from build123d import *

# Parameters (mm, degrees)
SKETCH2_W           = 86.2
SKETCH2_H           = 20
SKETCH2_R           = 7
BOSS_EXTRUDE1_DEPTH = 45
SKETCH3_R           = 1.375
CUT_EXTRUDE1_DEPTH  = 66.441653402
SKETCH4_R           = 4
CUT_EXTRUDE2_DEPTH  = 17
SKETCH5_R           = 7
SKETCH5_R_2         = 5
BOSS_EXTRUDE2_DEPTH = 21
SKETCH6_R           = 2
SKETCH6_R_2         = 2.5
CUT_EXTRUDE3_DEPTH  = 66.441653402
SKETCH7_R           = 5
CUT_EXTRUDE4_DEPTH  = 16
CUT_EXTRUDE5_REACH  = 67.442
SKETCH8_R           = 1
SKETCH9_W           = 60
SKETCH9_H           = 24.2
CUT_EXTRUDE6_DEPTH  = 66.441653471


with BuildPart() as part:
    # Sketch2 → Boss-Extrude1 (new, symmetric)
    with BuildSketch(Plane(origin=(0, 0, 0), x_dir=(0, 0, -1), z_dir=(1, 0, 0))):
        Rectangle(SKETCH2_W, SKETCH2_H)
        with Locations(Location((-24.1, 0, 0), (0, 0, 180))):
            Circle(SKETCH2_R, mode=Mode.SUBTRACT)
        with Locations(Location((24.1, 0, 0), (0, 0, 180))):
            Circle(SKETCH2_R, mode=Mode.SUBTRACT)
    extrude(amount=BOSS_EXTRUDE1_DEPTH, both=True)

    # Sketch3 → Cut-Extrude1 (cut, through all)
    with BuildSketch(Plane.XZ.offset(10)):
        with Locations(Location((-38.1, 36.195, 0), (0, 0, 270))):
            Circle(SKETCH3_R)
        with Locations(Location((38.1, 36.195, 0), (0, 0, 270))):
            Circle(SKETCH3_R)
        with Locations(Location((38.1, -36.195, 0), (0, 0, 270))):
            Circle(SKETCH3_R)
        with Locations(Location((-38.1, -36.195, 0), (0, 0, 270))):
            Circle(SKETCH3_R)
    extrude(amount=-CUT_EXTRUDE1_DEPTH, mode=Mode.SUBTRACT)

    # Sketch4 → Cut-Extrude2 (cut)
    with BuildSketch(Plane(origin=(0, 10, 0), x_dir=(1, 0, 0), z_dir=(0, 1, 0))):
        with Locations(Location((-38.1, -36.195, 0), (0, 0, 270))):
            Circle(SKETCH4_R)
        with Locations(Location((-38.1, 36.195, 0), (0, 0, 270))):
            Circle(SKETCH4_R)
        with Locations(Location((38.1, 36.195, 0), (0, 0, 270))):
            Circle(SKETCH4_R)
        with Locations(Location((38.1, -36.195, 0), (0, 0, 270))):
            Circle(SKETCH4_R)
    extrude(amount=-CUT_EXTRUDE2_DEPTH, mode=Mode.SUBTRACT)

    # Sketch5 → Boss-Extrude2 (add, symmetric)
    # profile 1 of 2: a face of its own
    with BuildSketch(Plane(origin=(0, 0, 0), x_dir=(0, 0, -1), z_dir=(1, 0, 0))):
        with Locations(Location((24.1, 0, 0), (0, 0, 180))):
            Circle(SKETCH5_R)
        with Locations(Location((24.1, 0, 0), (0, 0, 180))):
            Circle(SKETCH5_R_2, mode=Mode.SUBTRACT)
    # profile 2 of 2: a face of its own
    with BuildSketch(Plane(origin=(0, 0, 0), x_dir=(0, 0, -1), z_dir=(1, 0, 0))):
        with Locations(Location((-24.1, 0, 0), (0, 0, 180))):
            Circle(SKETCH5_R)
        with Locations(Location((-24.1, 0, 0), (0, 0, 180))):
            Circle(SKETCH5_R_2, mode=Mode.SUBTRACT)
    extrude(amount=BOSS_EXTRUDE2_DEPTH, both=True)

    # Sketch6 → Cut-Extrude3 (cut, through all)
    with BuildSketch(Plane(origin=(0, 10, 0), x_dir=(1, 0, 0), z_dir=(0, 1, 0))):
        with Locations(Location((30, 0, 0), (0, 0, 270))):
            Circle(SKETCH6_R)
        with Locations(Location((0, -36.195, 0), (0, 0, 270))):
            Circle(SKETCH6_R_2)
        with Locations(Location((0, 36.195, 0), (0, 0, 270))):
            Circle(SKETCH6_R_2)
    extrude(amount=-CUT_EXTRUDE3_DEPTH, mode=Mode.SUBTRACT)

    # Sketch7 → Cut-Extrude4 (cut)
    with BuildSketch(Plane.XZ.offset(10)):
        with Locations(Location((30, 0, 0), (0, 0, 270))):
            Circle(SKETCH7_R)
        with Locations(Location((0, 36.195, 0), (0, 0, 270))):
            Circle(SKETCH7_R)
        with Locations(Location((0, -36.195, 0), (0, 0, 270))):
            Circle(SKETCH7_R)
    extrude(amount=-CUT_EXTRUDE4_DEPTH, mode=Mode.SUBTRACT)

    # Sketch8 → Cut-Extrude5 (cut, up to next)
    with BuildSketch(Plane(origin=(0, 10, 0), x_dir=(1, 0, 0), z_dir=(0, 1, 0)), mode=Mode.PRIVATE) as cut_extrude5_sk1:
        with Locations(Location((35, -24.1, 0), (0, 0, 270))):
            Circle(SKETCH8_R)
    cut_extrude5_tool1 = extrude(cut_extrude5_sk1.sketch, amount=-CUT_EXTRUDE5_REACH, mode=Mode.PRIVATE) & part.part
    # Sketch8 → Cut-Extrude5 (cut, up to next)
    with BuildSketch(Plane(origin=(0, 10, 0), x_dir=(1, 0, 0), z_dir=(0, 1, 0)), mode=Mode.PRIVATE) as cut_extrude5_sk2:
        with Locations(Location((-35, -24.1, 0), (0, 0, 270))):
            Circle(SKETCH8_R)
    cut_extrude5_tool2 = extrude(cut_extrude5_sk2.sketch, amount=-CUT_EXTRUDE5_REACH, mode=Mode.PRIVATE) & part.part
    # Sketch8 → Cut-Extrude5 (cut, up to next)
    with BuildSketch(Plane(origin=(0, 10, 0), x_dir=(1, 0, 0), z_dir=(0, 1, 0)), mode=Mode.PRIVATE) as cut_extrude5_sk3:
        with Locations(Location((-35, 24.1, 0), (0, 0, 270))):
            Circle(SKETCH8_R)
    cut_extrude5_tool3 = extrude(cut_extrude5_sk3.sketch, amount=-CUT_EXTRUDE5_REACH, mode=Mode.PRIVATE) & part.part
    # Sketch8 → Cut-Extrude5 (cut, up to next)
    with BuildSketch(Plane(origin=(0, 10, 0), x_dir=(1, 0, 0), z_dir=(0, 1, 0)), mode=Mode.PRIVATE) as cut_extrude5_sk4:
        with Locations(Location((35, 24.1, 0), (0, 0, 270))):
            Circle(SKETCH8_R)
    cut_extrude5_tool4 = extrude(cut_extrude5_sk4.sketch, amount=-CUT_EXTRUDE5_REACH, mode=Mode.PRIVATE) & part.part
    add(cut_extrude5_tool1.solids().sort_by_distance((35, 10, 24.1))[0], mode=Mode.SUBTRACT)
    add(cut_extrude5_tool2.solids().sort_by_distance((-35, 10, 24.1))[0], mode=Mode.SUBTRACT)
    add(cut_extrude5_tool3.solids().sort_by_distance((-35, 10, -24.1))[0], mode=Mode.SUBTRACT)
    add(cut_extrude5_tool4.solids().sort_by_distance((35, 10, -24.1))[0], mode=Mode.SUBTRACT)

    # Sketch9 → Cut-Extrude6 (cut, through all)
    with BuildSketch(Plane(origin=(0, 10, 0), x_dir=(1, 0, 0), z_dir=(0, 1, 0))):
        with Locations((-10, 0)):
            Rectangle(SKETCH9_W, SKETCH9_H)
    extrude(amount=-CUT_EXTRUDE6_DEPTH, mode=Mode.SUBTRACT)


solid = part.part
Check sheet for the modelled part. Datum: model origin and axes. Units: mm. A direction names the side the tool comes from. Give positions to 0.01 mm unless a question says otherwise; leave off trailing zeros. Loops run counter-clockwise (first coordinate to the right, second up) from the corner with the lowest first, then second, coordinate; pieces in that order, holes last. Notation, with made-up numbers: M 52.25,24.5 L 84.25,24.5 A21 ccw 84.25,42.5 Z; hole C 28.5,-28 d4. An arc over 180 degrees is marked long. Use a Markdown table: item, result. Add a question column.
Q1. Sectioned sample at C-C, the plane z = -9. Record the cut outline in (x, y).
Q2. Sectioned sample at B-B, the plane x = 38.1. Record the cut outline in (y, z) (3 decimals).
Q3. Sectioned sample at D-D, the plane y = 0. Give the number of separate pieces and of enclosed holes in the cut face, then the cut area to 3 significant figures.
Q4. Sectioned sample at A-A, the plane x = -30.5. Record the cut outline in (y, z).
Q5. Mould release check, pull along Z, two halves, no side actions. Record for faces 1 (the cylindrical face through (39.463, -8.521, 36.374)), 2 (the flat face through (1, 0, 43.1)), 3 (the flat face through (1, 0, -43.1)): pulls with the +Z half, pulls with the -Z half, needs draft (parallel to the pull), parting line crosses it, or undercut.
Q6. Go/stop test with flat-tipped pins: pin 1 (2.5 mm diameter, centred on x = 38.1, z = -36.195, fed in from +Y); pin 2 (5 mm diameter, centred on x = -1, z = 35, fed in from -Y). Record where each tip stops, or that it passes through.
Q7. Scan lines: line 1 along X through (y, z) = (7.55, 24.1); line 2 along Y through (x, z) = (-10, -24); line 3 along X through (y, z) = (-0.75, 6). Record each from-to range of solid material in increasing order. Write a range as [from, to].
Q8. Tool access check on faces 4 (the flat face through (-38, -7, -34)), 5 (the cylindrical face through (-3.042, -2.112, 40.163)), 6 (the flat face through (21, 10, 1)), 7 (the flat face through (-10, 0, 12.1)). Record the directions out of +Z, -Z, +X, -X, +Y, -Y that give a thin tool (end or side, any length) a straight path to the whole face; none if there is none.
Verdict:
| question | item | result |
|---|---|---|
| 1 | outline | M -45,-10 L -40,-10 L -40,10 L -45,10 Z; M 20,-10 L 45,-10 L 45,10 L 20,10 Z |
| 2 | outline | M -10,-43.1 L 10,-43.1 L 10,-40.195 L -7,-40.195 L -7,-37.57 L -10,-37.57 Z; M -10,-34.82 L -7,-34.82 L -7,-32.195 L 10,-32.195 L 10,32.195 L -7,32.195 L -7,34.82 L -10,34.82 Z; M -10,37.57 L -7,37.57 L -7,40.195 L 10,40.195 L 10,43.1 L -10,43.1 Z; hole C 0,-24.1 d14; hole C 0,24.1 d14 |
| 3 | separate pieces | 3 |
| 3 | enclosed holes | 8 |
| 3 | area | 3,690 mm^2 |
| 4 | outline | M -10,-43.1 L 10,-43.1 L 10,-12.1 L -10,-12.1 Z; M -10,12.1 L 10,12.1 L 10,43.1 L -10,43.1 Z; hole C 0,-24.1 d14; hole C 0,24.1 d14 |
| 5 | face 1 | undercut |
| 5 | face 2 | pulls with the +Z half |
| 5 | face 3 | pulls with the -Z half |
| 6 | pin 1 | through |
| 6 | pin 2 | y = 6 |
| 7 | line 1 | [-45, -36], [-34, 34], [36, 45] |
| 7 | line 2 | [-10, -5], [5, 10] |
| 7 | line 3 | [-45, -40], [20, 45] |
| 8 | face 4 | +Y |
| 8 | face 5 | -Y |
| 8 | face 6 | +Z, -Z, +X, -X, +Y |
| 8 | face 7 | +Y, -Y |
